The figure shows three views and two pictorial views of one solid part (mm, origin at its lowest corner). Answer the questions. A direction names the side the tool comes from. Round coordinates to 2 decimals unless told otherwise and drop trailing zeros. Order: outer loops, then holes, each group sorted by start corner. A loop starts at its lowest first (then second) coordinate and runs counter-clockwise, first axis right, second up. Notation, with made-up numbers: (83.25, 39.25) - (136.25, 39.25) arc R28 cw to (136.25, 75.25) - close; hole circle Ø5 at (54.5, 19.25). An arc over 180 degrees is marked (long way). Use CSV: the item, a comma, the result in double quotes.
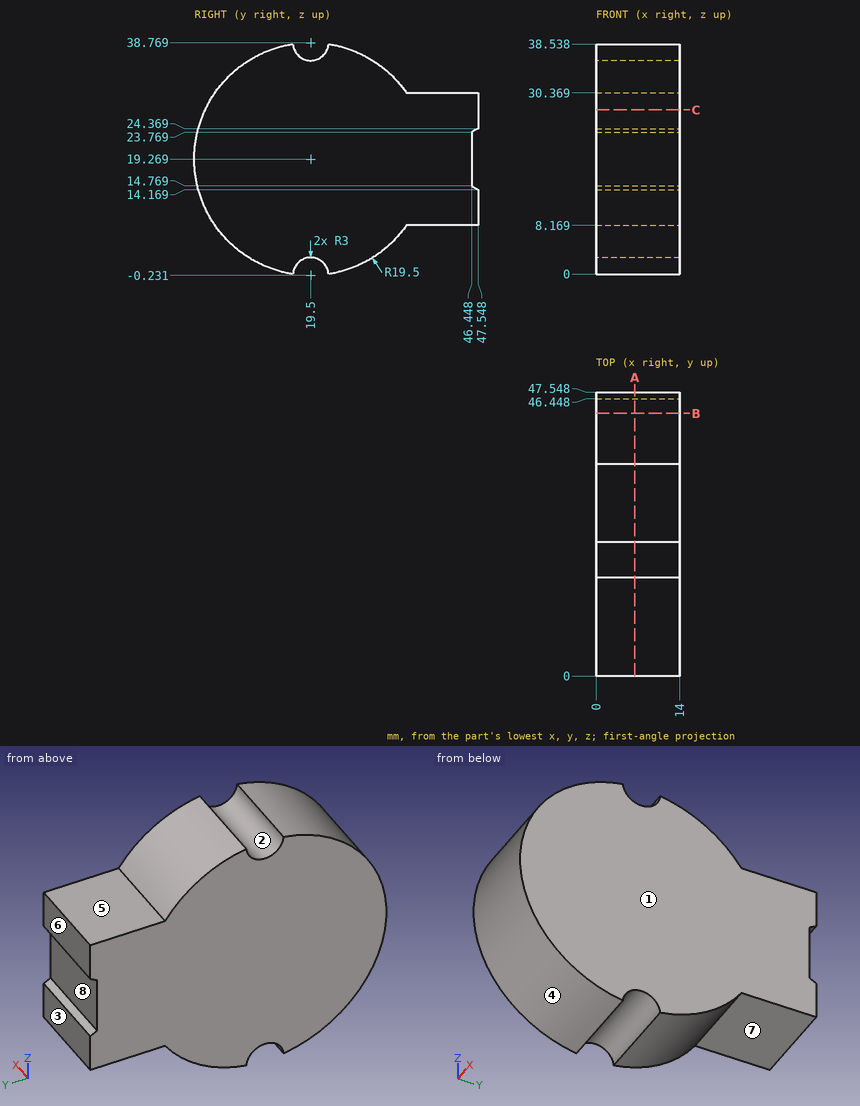
(1) The mould has two halves that part along Y. Classify the marked faces 1, 2 and 3: released by +Y, released by -Y, zero draft, split by the parting line, or undercut.
Findings below:
face 1,"zero draft"
face 2,"undercut"
face 3,"released by +Y"
(2) Find section C-C (z = 27.5). Determine the outline of the cut face in (x, y), and give its area (3 significant figures).
Findings below:
outline,"(0, 1.82) - (14, 1.82) - (14, 47.55) - (0, 47.55) - close"
area,"640 mm²"
(3) Each of these flat-tipped pins is pushed along its axis until it touches: pin 1 (3 mm diameter, centred on x = 8.5, y = 12, fed in from +Z); pin 2 (1 mm diameter, centred on x = 6.5, z = 15.5, fed in from -Y); pin 3 (7 mm diameter, centred on x = 9.5, z = 17.5, fed in from +Y); pin 4 (1.5 mm diameter, centred on x = 9, y = 36.5, fed in from -Z). Where does it stop, or does it pass through?
Findings below:
pin 1,"stops at z = 37.82"
pin 2,"stops at y = 0.28"
pin 3,"stops at y = 47.55"
pin 4,"stops at z = 8.17"
(4) Find the intervals of material crossed by L1, parallel to Y at x = 3, z = 10.5; L2, parallel to Y at x = 2.5, z = 7 (1 decimal); L3, parallel to Z at x = 3.25, y = 5.5 (1 decimal), in increasing order. Write a range as from..to.
Findings below:
L1,"y = 2.08..47.55"
L2,"y = 4.3..34.7"
L3,"z = 5.7..32.8"
(5) For the marked faces 4, 5, 6, 7 and 8, determine the directions among +Z, -Z, +X, -X, +Y, -Y from which every point of the face is accessible in a straight line to the end or side of a thin tool.
Findings below:
face 4,"+X, -X, -Y"
face 5,"+Z, +X, -X, +Y"
face 6,"+Z, -Z, +X, -X, +Y"
face 7,"-Z, +X, -X, +Y"
face 8,"+X, -X, +Y"
(6) Find section B-B (y = 44). Determine the outline of the cut face in (x, z).
Findings below:
outline,"(0, 8.17) - (14, 8.17) - (14, 30.37) - (0, 30.37) - close"
(7) Find section A-A (x = 6.5). Determine the outline of the cut face in (y, z), and give its area (3 significant figures).
Findings below:
outline,"(16.51, 0) arc R3 cw to (22.49, 0) arc R19.5 ccw to (35.53, 8.17) - (47.55, 8.17) - (47.55, 14.17) - (46.45, 14.77) - (46.45, 23.77) - (47.55, 24.37) - (47.55, 30.37) - (35.53, 30.37) arc R19.5 ccw to (22.49, 38.54) arc R3 cw to (16.51, 38.54) arc R19.5 ccw to start"
area,"1,370 mm²"
